Geometry: final body of the model. Coordinates: model frame, mm. Face numbers are marked on the shaded views. A direction names the side the tool comes from. Round coordinates to 2 decimals unless told otherwise and drop trailing zeros. Loops run counter-clockwise (first coordinate to the right, second up) from the corner with the lowest first, then second, coordinate; pieces in that order, holes last. Notation, with made-up numbers: (19.5, 27) -> (47.5, 27) arc R36 cw to (47.5, 62) -> close; hole circle Ø4 at (66.25, 49). An arc over 180 degrees is marked (long way). Answer in a Markdown table with one row per item.
```python
from build123d import *

# Parameters (mm, degrees)
ENL_V_MAT_EXTRU_1_DEPTH = 5
ENL_V_MAT_EXTRU_2_REACH = 45.997
ESQUISSE3_W             = 0.6
ESQUISSE3_H             = 14


with BuildPart() as part:
    # Esquisse1 → Révolution1 (revolve)
    with BuildSketch(Plane.XY):
        Polygon((0, 33.5), (-11, 33.5), (-14, 32.5), (-14, 31), (-10.85, 31), (-10.85, 17), (-9.985, 17), (-9.985, 10), (-6, 6), (-6, 0), (0, 0), align=None)
    revolve(axis=Axis((0, 33.5, 0), (0, -1, 0)))

    # Esquisse2 → Enlèv. mat.-Extru.1 (cut)
    with BuildSketch(Plane(origin=(0, 33.5, 0), x_dir=(1, 0, 0), z_dir=(0, 1, 0))):
        Polygon((-3.45, 0.9), (3.45, 0.9), (3.45, 0), (2.5, -0.95), (-2.5, -0.95), (-3.45, 0), align=None)
    extrude(amount=-ENL_V_MAT_EXTRU_1_DEPTH, mode=Mode.SUBTRACT)

    # Esquisse3 → Enlèv. mat.-Extru.2 (cut, up to next)
    with BuildSketch(Plane(origin=(0, 0, -10.85), x_dir=(-1, 0, 0), z_dir=(0, 0, -1)), mode=Mode.PRIVATE) as enl_v_mat_extru_2_sk1:
        with Locations((10.55, 24)):
            Rectangle(ESQUISSE3_W, ESQUISSE3_H)
    enl_v_mat_extru_2_tool1 = extrude(enl_v_mat_extru_2_sk1.sketch, amount=-ENL_V_MAT_EXTRU_2_REACH, mode=Mode.PRIVATE) & part.part
    # Esquisse3 → Enlèv. mat.-Extru.2 (cut, up to next)
    with BuildSketch(Plane(origin=(0, 0, -10.85), x_dir=(-1, 0, 0), z_dir=(0, 0, -1)), mode=Mode.PRIVATE) as enl_v_mat_extru_2_sk2:
        with Locations((-10.55, 24)):
            Rectangle(ESQUISSE3_W, ESQUISSE3_H)
    enl_v_mat_extru_2_tool2 = extrude(enl_v_mat_extru_2_sk2.sketch, amount=-ENL_V_MAT_EXTRU_2_REACH, mode=Mode.PRIVATE) & part.part
    add(enl_v_mat_extru_2_tool1.solids().sort_by_distance((-10.55, 24, -10.85))[0], mode=Mode.SUBTRACT)
    add(enl_v_mat_extru_2_tool2.solids().sort_by_distance((10.55, 24, -10.85))[0], mode=Mode.SUBTRACT)


solid = part.part
```
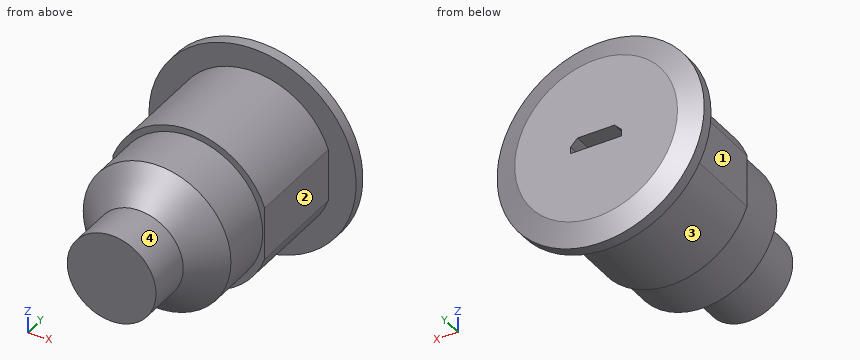
Item 1: Pin query (flat end, axial travel): pin 1 Ø5 at (y, z) = (30, -8) entering from -X; pin 2 Ø8 at (x, y) = (5.5, 7) entering from +Z; pin 3 Ø1.5 at (y, z) = (17, 5.5) entering from +X (3 decimals). Return the tip coordinate at first contact, or that it passes through.
Answer:
| item | result |
|---|---|
| pin 1 | stops at x = -12.78 |
| pin 2 | stops at z = 9.57 |
| pin 3 | stops at x = 9.755 |
Item 2: Cut plane D-D (y = 26). Output: boundary loops of the cut face in (x, z), then the cut area to 3 significant figures.
Answer:
| item | result |
|---|---|
| outline | (-10.25, -3.56) arc R10.85 ccw to (10.25, -3.56) -> (10.25, 3.56) arc R10.85 ccw to (-10.25, 3.56) -> close |
| area | 364 mm² |
Item 3: Line query: probe 1 along X at (y, z) = (15, -0.25); probe 2 along Y at (x, z) = (2.5, -10.25); probe 3 along X at (y, z) = (16, -6). Output: solid intervals per line, ascending. Write a range as [from, to].
Answer:
| item | result |
|---|---|
| probe 1 | x = [-9.98, 9.98] |
| probe 2 | y = [17, 33.5] |
| probe 3 | x = [-7.98, 7.98] |
Item 4: Cut plane B-B (x = 0). Output: boundary loops of the cut face in (y, z) (3 decimals), then the cut area to 3 significant figures.
Answer:
| item | result |
|---|---|
| outline | (0, -6) -> (6, -6) -> (10, -9.985) -> (17, -9.985) -> (17, -10.85) -> (31, -10.85) -> (31, -14) -> (32.5, -14) -> (33.5, -11) -> (33.5, -0.9) -> (28.5, -0.9) -> (28.5, 0.95) -> (33.5, 0.95) -> (33.5, 11) -> (32.5, 14) -> (31, 14) -> (31, 10.85) -> (17, 10.85) -> (17, 9.985) -> (10, 9.985) -> (6, 6) -> (0, 6) -> close |
| area | 637 mm² |
Item 5: Cut plane C-C (y = 13.5). Output: boundary loops of the cut face in (x, z) (3 decimals).
Answer:
| item | result |
|---|---|
| outline | circle Ø19.97 at (0, 0) |
Item 6: Reachability of the marked faces 1, 2, 3 and 4 from +Z, -Z, +X, -X, +Y, -Y: full face, straight path, thin tool, end or side. Return the list, or none.
Answer:
| item | result |
|---|---|
| face 1 | +Z, -Z, -X, -Y |
| face 2 | +Z, -Z, +X, -Y |
| face 3 | -Z, -Y |
| face 4 | -Y |
Item 7: Cut plane A-A (y = 30.5). Output: boundary loops of the cut face in (x, z).
Answer:
| item | result |
|---|---|
| outline | (-10.25, -3.56) arc R10.85 ccw to (10.25, -3.56) -> (10.25, 3.56) arc R10.85 ccw to (-10.25, 3.56) -> close; hole (-3.45, -0.9) -> (3.45, -0.9) -> (3.45, 0) -> (2.5, 0.95) -> (-2.5, 0.95) -> (-3.45, 0) -> close |
